Can you work these out from the model? Positions are in its coordinate system, mm. Face numbers are marked on the shaded views. A direction names the side the tool comes from. Give positions to 0.01 mm unless a question says otherwise; leave off trailing zeros. Write each loop counter-clockwise with the first axis right and the second up, starting at its lowest first coordinate (ties: lowest second). Pieces come first, ordered by that corner, then holes.
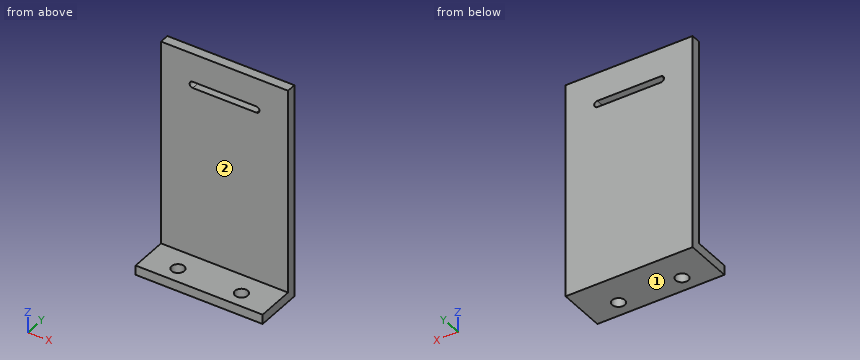
from build123d import *

# Parameters (mm, degrees)
SKETCH1_W           = 40
SKETCH1_H           = 15
SKETCH1_R           = 2
BOSS_EXTRUDE1_DEPTH = 3
SKETCH2_W           = 40
SKETCH2_H           = 3
BOSS_EXTRUDE2_DEPTH = 65
CUT_EXTRUDE1_DEPTH  = 65


with BuildPart() as part:
    # Sketch1 → Boss-Extrude1 (new body)
    with BuildSketch(Plane.XY):
        Rectangle(SKETCH1_W, SKETCH1_H)
        with Locations((-10, -2.5)):
            Circle(SKETCH1_R, mode=Mode.SUBTRACT)
        with Locations((10, -2.5)):
            Circle(SKETCH1_R, mode=Mode.SUBTRACT)
    extrude(amount=BOSS_EXTRUDE1_DEPTH)

    # Sketch2 → Boss-Extrude2 (add)
    with BuildSketch(Plane.XY.offset(3)):
        with Locations((0, 6)):
            Rectangle(SKETCH2_W, SKETCH2_H)
    extrude(amount=BOSS_EXTRUDE2_DEPTH)

    # Sketch3 → Cut-Extrude1 (cut)
    with BuildSketch(Plane.XZ.offset(-4.5)):
        with BuildLine():
            Line((-10, 59), (10, 59))
            ThreePointArc((10, 59), (11, 58), (10, 57))
            Line((10, 57), (-10, 57))
            ThreePointArc((-10, 57), (-11, 58), (-10, 59))
        make_face()
    extrude(amount=-CUT_EXTRUDE1_DEPTH, mode=Mode.SUBTRACT)


solid = part.part
(1) If I drill on L1, parallel to Y at x = 10, z = 1; L2, parallel to Z at x = 0.5, y = 5; L3, parallel to Z at x = -12.5, y = 2, over which ranges is the centre line in solid material (lowest first)?
Returned:
L1: y = -7.5 to -4.5, -0.5 to 7.5
L2: z = 0 to 57, 59 to 68
L3: z = 0 to 3
(2) Imagine slicing it at B-B, the plane x = -0.5. Write out the boundary of the cut face in (y, z), plus the area to 3 significant figures.
Returned:
outline: (-7.5, 0) - (7.5, 0) - (7.5, 57) - (4.5, 57) - (4.5, 3) - (-7.5, 3) - close; (4.5, 59) - (7.5, 59) - (7.5, 68) - (4.5, 68) - close
area: 234 mm2
(3) For the marked faces 1 and 2, which set-ups out of +Z, -Z, +X, -X, +Y, -Y let a thin tool reach every point of the face, with its end or its side?
Returned:
face 1: -Z, +X, -X, +Y, -Y
face 2: +Z, +X, -X, -Y
(4) Imagine slicing it at A-A, the plane y = -2.5. Write out the boundary of the cut face in (x, z).
Returned:
outline: (-20, 0) - (-12, 0) - (-12, 3) - (-20, 3) - close; (-8, 0) - (8, 0) - (8, 3) - (-8, 3) - close; (12, 0) - (20, 0) - (20, 3) - (12, 3) - close
(5) Imagine slicing it at C-C, the plane z = 58. Write out the boundary of the cut face in (x, y), plus the area to 3 significant figures.
Returned:
outline: (-20, 4.5) - (-11, 4.5) - (-11, 7.5) - (-20, 7.5) - close; (11, 4.5) - (20, 4.5) - (20, 7.5) - (11, 7.5) - close
area: 54.0 mm2
(6) Imagine slicing it at D-D, the plane z = 13.5. Write out the boundary of the cut face in (x, y).
Returned:
outline: (-20, 4.5) - (20, 4.5) - (20, 7.5) - (-20, 7.5) - close
(7) Will these pins go through, and if not, where does the flat tip stop? P1, Ø12, axis at x = -14, z = 45.5, coming from the -Y side; P2, Ø3.5, axis at x = -2.5, y = -3.5, coming from the +Z side; P3, Ø0.9, axis at x = -0.5, y = 5.5, coming from the -Z side.
Returned:
P1: stops at y = 4.5
P2: stops at z = 3
P3: stops at z = 0
